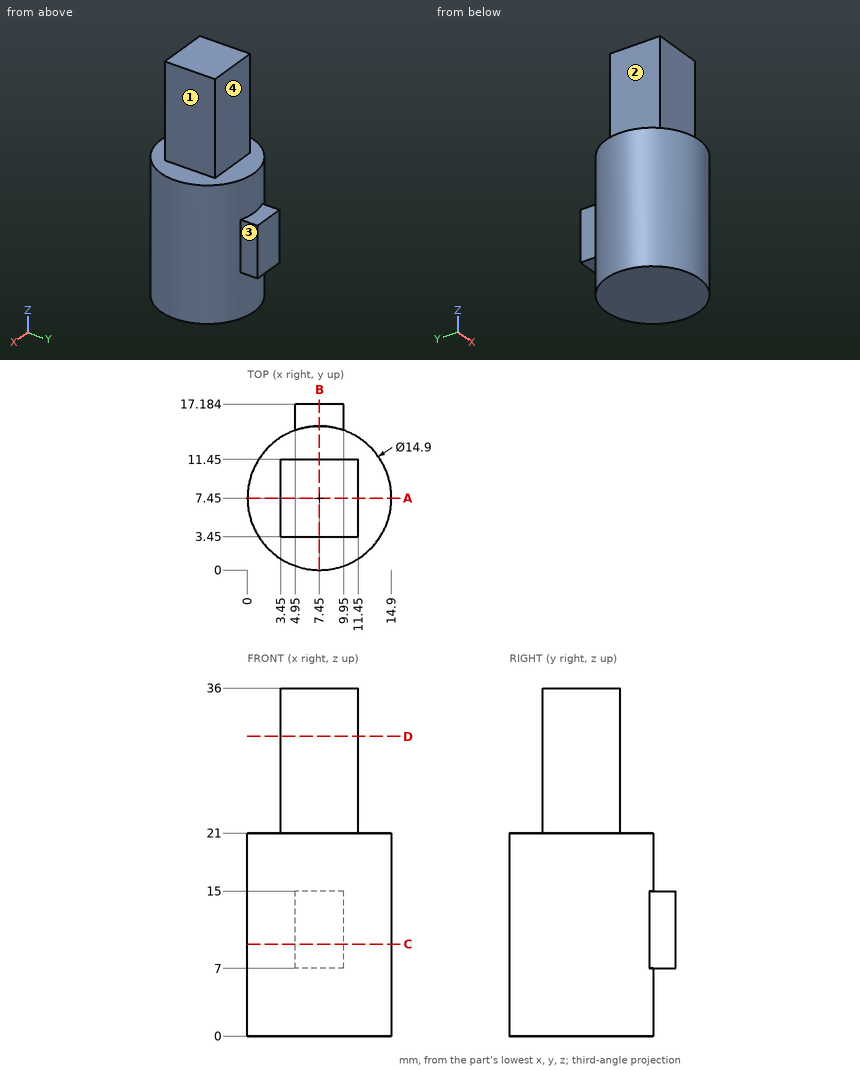
The drawing under review shows one solid part. Ordinate dimensions are in mm from its lowest x, y, z. A direction names the side the tool comes from. Give positions to 0.01 mm unless a question says otherwise; leave off trailing zeros. Write each loop counter-clockwise with the first axis right and the second up, starting at its lowest first coordinate (ties: lowest second). Pieces come first, ordered by that corner, then holes.
1. Tool access review of the marked faces 1, 2, 3 and 4: name each direction out of +Z, -Z, +X, -X, +Y, -Y from which nothing blocks a thin tool from reaching the whole face with its end or side.
2. For P1, Ø1.4, axis at x = 8, y = 16, coming from the +Z side; P2, Ø4, axis at x = 7.5, z = 25, coming from the -Y side; P3, Ø4, axis at x = 3, z = 22, coming from the -Y side, all flat-tipped, find the tip position at first contact; note any pin that passes through.
3. Add section C-C, the plane z = 9.5. Write out the cut boundary in (x, y).
4. Add section D-D, the plane z = 31. Write out the cut boundary in (x, y).
5. Wall thickness on L1, parallel to X at y = 7.25, z = 16; L2, parallel to Z at x = 1.25, y = 4.5; L3, parallel to X at y = 5.5, z = 26.5: over which ranges is each line inside the solid? List them lowest first.
6. Add section B-B, the plane x = 7.45. Write out the cut boundary in (y, z), plus the area to 3 significant figures.
7. Add section A-A, the plane y = 7.45. Write out the cut boundary in (x, z).
Worked answers:
1. face 1: +Z, +X, +Y, -Y
1. face 2: +Z, -X, +Y, -Y
1. face 3: +Z, -Z, +X, +Y
1. face 4: +Z, +X, -X, +Y
2. P1: stops at z = 15
2. P2: stops at y = 3.45
2. P3: stops at y = 0.51
3. outline: (4.95, 14.47) arc R7.45 ccw (long way) to (9.95, 14.47) - (9.95, 17.18) - (4.95, 17.18) - close
4. outline: (3.45, 3.45) - (11.45, 3.45) - (11.45, 11.45) - (3.45, 11.45) - close
5. L1: x = 0 to 14.9
5. L2: z = 0 to 21
5. L3: x = 3.45 to 11.45
6. outline: (0, 0) - (14.9, 0) - (14.9, 7) - (17.18, 7) - (17.18, 15) - (14.9, 15) - (14.9, 21) - (11.45, 21) - (11.45, 36) - (3.45, 36) - (3.45, 21) - (0, 21) - close
6. area: 451 mm2
7. outline: (0, 0) - (14.9, 0) - (14.9, 21) - (11.45, 21) - (11.45, 36) - (3.45, 36) - (3.45, 21) - (0, 21) - close
